Build history of the part. All positions in model axes, mm. A direction names the side the tool comes from. Give positions to 0.01 mm unless a question says otherwise; leave off trailing zeros. Order: outer loops, then holes, each group sorted by start corner. A loop starts at its lowest first (then second) coordinate and runs counter-clockwise, first axis right, second up. Notation, with made-up numbers: (41.25, -20) - (87.25, -20) arc R16 ccw to (87.25, 4) - close; hole circle Ø3 at (-18.75, 47.25). An arc over 180 degrees is marked (long way). One line per item, written item: value.
```python
from build123d import *

# Parameters (mm, degrees)
SALIENTE_EXTRUIR1_DEPTH = 20
REDONDEO1_R             = 20
CROQUIS3_W              = 20
CROQUIS3_H              = 22.736865604
CROQUIS3_H_2            = 22.452131832
CORTAR_EXTRUIR2_DEPTH   = 10


with BuildPart() as part:
    # Croquis1 → Saliente-Extruir1 (new body)
    with BuildSketch(Plane(origin=(0, 0, 0), x_dir=(1, 0, 0), z_dir=(0, 1, 0))):
        Polygon((-70, 0), (-50, 0), (50, -55), (70, -55), (70, -75), (50, -75), (-50, -20), (-70, -20), align=None)
    extrude(amount=SALIENTE_EXTRUIR1_DEPTH)

    # Redondeo1
    redondeo1_edges = [part.edges().sort_by_distance(p)[0] for p in [
        (-50, 10, 0),
        (50, 10, 55),
        (50, 10, 75),
        (-50, 10, 20),
    ]]
    fillet(redondeo1_edges, radius=REDONDEO1_R)

    # Croquis3 → Cortar-Extruir2 (cut)
    with BuildSketch(Plane(origin=(0, 0, 0), x_dir=(1, 0, 0), z_dir=(0, 1, 0))):
        with Locations((-60, -11.368432802)):
            Rectangle(CROQUIS3_W, CROQUIS3_H)
        with Locations((60, -63.773934084)):
            Rectangle(CROQUIS3_W, CROQUIS3_H_2)
    extrude(amount=CORTAR_EXTRUIR2_DEPTH, mode=Mode.SUBTRACT)


solid = part.part
```
(1) 3-axis set-ups, long thin cutter, end or side, ignore diameter. For faces 1 (the face through (-62, 15, 20)), 2 (the face through (50, 5, 64)), 3 (the face through (62, 15, 55)), 4 (the face through (-60, 10, 10)): which of +Z, -Z, +X, -X, +Y, -Y reach the whole face in a straight line?
Completed:
face 1: +Z, -X, +Y, -Y
face 2: +Z, -Z, +X, -Y
face 3: -Z, +X, +Y, -Y
face 4: +Z, -Z, -X, -Y
(2) Slice it at B-B, the plane z = 11. Give the cut face in (x, y), and give its area (3 significant figures).
Completed:
outline: (-70, 10) - (-50, 10) - (-50, 0) - (-30, 0) - (-30, 20) - (-70, 20) - close
area: 600 mm²
(3) Slice it at C-C, the plane x = 25. Give the cut face in (y, z).
Completed:
outline: (0, 41.25) - (20, 41.25) - (20, 61.25) - (0, 61.25) - close
(4) Pin check, flat tips, straight feed: P1, Ø2, axis at y = 17.5, z = 37.5, coming from the +X side; P2, Ø22, axis at x = 59.5, z = 61.5, coming from the -Y side; P3, Ø1, axis at x = -45.5, y = 17.5, coming from the -Z side; P4, Ø5, axis at x = 61, y = 14.5, coming from the -Z side. Stop position of each tip, or through.
Completed:
P1: x = 20
P2: y = 0
P3: z = 2.21
P4: z = 55
(5) Slice it at A-A, the plane y = 12.25. Give the cut face in (x, z), and give its area (3 significant figures).
Completed:
outline: (-70, 0) - (-55.14, 0) arc R20 ccw to (-45.5, 2.48) - (45.5, 52.52) arc R20 cw to (55.14, 55) - (70, 55) - (70, 75) - (55.14, 75) arc R20 ccw to (45.5, 72.52) - (-45.5, 22.48) arc R20 cw to (-55.14, 20) - (-70, 20) - close
area: 2,800 mm²
(6) Slice it at D-D, the plane y = 1.5. Give the cut face in (x, z).
Completed:
outline: (-50, 0.67) arc R20 ccw to (-45.5, 2.48) - (45.5, 52.52) arc R20 cw to (50, 54.33) - (50, 74.33) arc R20 ccw to (45.5, 72.52) - (-45.5, 22.48) arc R20 cw to (-50, 20.67) - close
(7) Drill centre lines: line 1 (Y direction, x = -55.5, z = 13.5); line 2 (X direction, y = 12, z = 5.5); line 3 (Z direction, x = -61, y = 14.75). Where is each one in solid material? Low to high.
Completed:
line 1: 10 to 20
line 2: -70 to -40
line 3: 0 to 20
